from build123d import *

# Parameters (mm, degrees)
F1_DEPTH = 50.8


with BuildPart() as f1:
    # F0 (on Front) → F1 (new body)
    with BuildSketch(Plane.XZ):
        with BuildLine():
            ThreePointArc((24.8326570204, -5.338459076), (25.2577660168, -2.6842607624), (25.4, 0))
            ThreePointArc((25.4, 0), (23.1920807644, 10.3579626287), (16.9521740302, 18.9151736881))
            ThreePointArc((16.9521740302, 18.9151736881), (14.9297454082, 20.5490316571), (12.750889326, 21.9675856979))
            ThreePointArc((12.750889326, 21.9675856979), (0, 25.4), (-12.750889326, 21.9675856979))
            ThreePointArc((-12.750889326, 21.9675856979), (-14.9297454082, 20.5490316571), (-16.9521740302, 18.9151736881))
            ThreePointArc((-16.9521740302, 18.9151736881), (-24.1568355139, 7.8490316571), (-24.8326570204, -5.338459076))
            ThreePointArc((-24.8326570204, -5.338459076), (-24.1568355139, -7.8490316571), (-23.2279090598, -10.2773654556))
            ThreePointArc((-23.2279090598, -10.2773654556), (-14.9297454082, -20.5490316571), (-2.5965367436, -25.2669348545))
            ThreePointArc((-2.5965367436, -25.2669348545), (0, -25.4), (2.5965367436, -25.2669348545))
            ThreePointArc((2.5965367436, -25.2669348545), (14.9297454082, -20.5490316571), (23.2279090598, -10.2773654556))
            ThreePointArc((23.2279090598, -10.2773654556), (24.1568355139, -7.8490316571), (24.8326570204, -5.338459076))
        make_face()
    extrude(amount=F1_DEPTH)


solid = f1.part
Could you check a few things on this model? Use its own coordinates, in mm. Give positions to 0.01 mm unless a question says otherwise; leave off trailing zeros. Order: outer loops, then holes, each group sorted by start corner. A loop starts at its lowest first (then second) coordinate and runs counter-clockwise, first axis right, second up. Notation, with made-up numbers: (51, -24.5) -> (103, -24.5) arc R6 cw to (103, -15.5) -> close; hole circle Ø7 at (-16.5, -25). An arc over 180 degrees is marked (long way). Answer in a Markdown table with one row per item. Add a question column.
Item 1: I'm going to push flat-ended pins straight in: P1, Ø3, axis at x = 3, y = -44, coming from the +Z side; P2, Ø3, axis at y = -5.5, z = 6.5, coming from the -X side; P3, Ø2, axis at x = 13, y = -19.5, coming from the -Z side; P4, Ø12, axis at y = -39, z = -5, coming from the -X side. Where does each tip first touch, or does it pass through?
Item 2: Imagine slicing it at C-C (z = 16). List the corners of the cut face in (x, y) for me.
Item 3: Please list where these lines run through material, in increasing order: probe 1 along Z at (x, y) = (15, -18); probe 2 along X at (y, z) = (-17, 4.5); probe 3 along X at (y, z) = (-24, -5.5).
Item 4: Imagine slicing it at B-B (x = -7). List the corners of the cut face in (y, z) for me, and give its area (3 significant figures).
Item 5: Imagine slicing it at A-A (y = -45). List the corners of the cut face in (x, z) for me.
Result:
| question | item | result |
|---|---|---|
| 1 | P1 | z = 25.36 |
| 1 | P2 | x = -24.9 |
| 1 | P3 | z = -22.39 |
| 1 | P4 | x = -25.4 |
| 2 | outline | (-19.73, -50.8) -> (19.73, -50.8) -> (19.73, 0) -> (-19.73, 0) -> close |
| 3 | probe 1 | -20.5 to 20.5 |
| 3 | probe 2 | -25 to 25 |
| 3 | probe 3 | -24.8 to 24.8 |
| 4 | outline | (-50.8, -24.42) -> (0, -24.42) -> (0, 24.42) -> (-50.8, 24.42) -> close |
| 4 | area | 2,480 mm2 |
| 5 | outline | circle Ø50.8 at (0, 0) |
